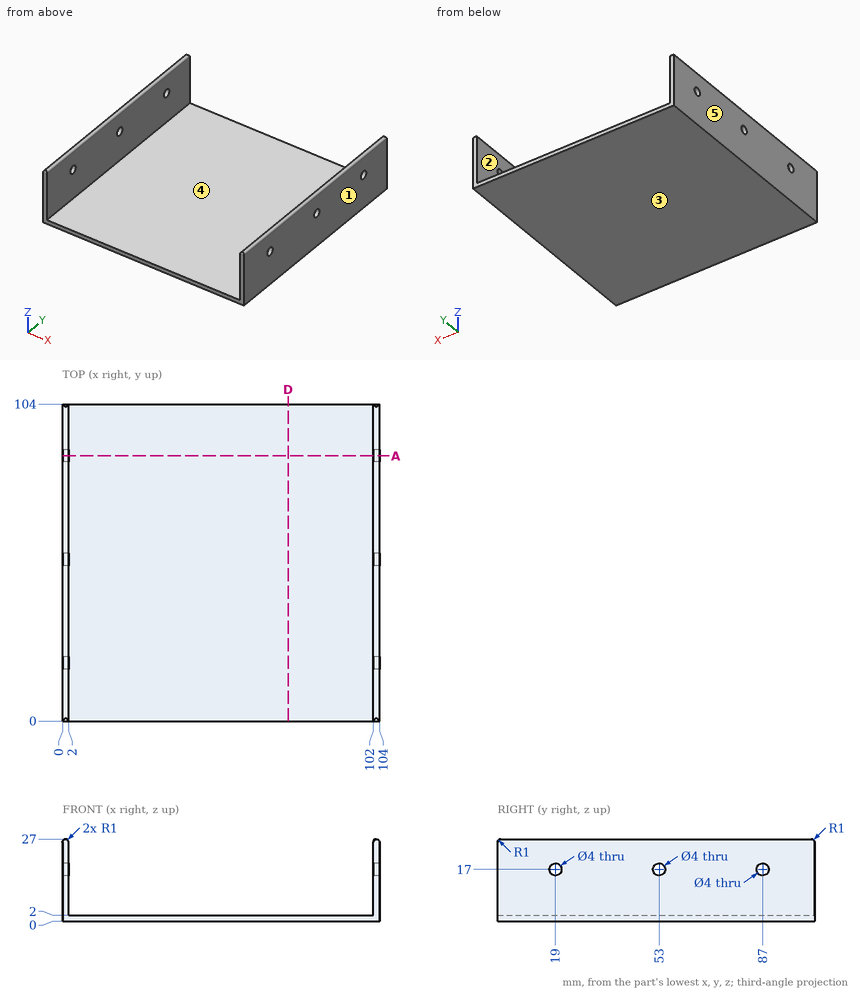
Answer from the drawing. Dimensions are ordinates in mm from the lowest x, y and z of the part. A direction names the side the tool comes from. Coordinates: 2 decimals unless noted, no trailing zeros. Write each loop counter-clockwise with the first axis right and the second up, starting at its lowest first coordinate (ties: lowest second). Pieces come first, ordered by that corner, then holes. Notation, with made-up numbers: (48.5, -39.5) - (92.5, -39.5) arc R24 cw to (92.5, -13.5) - close; hole circle Ø2 at (17.5, 65). An arc over 180 degrees is marked (long way). Return JSON: item names as keys, results as strings. Group by question number.
Q1. For a pull along X with two mould halves and no side action, classify the marked faces 3, 4 and 5 as +X half, -X half, draft (parallel to the pull), parting line (faces both ways), or undercut.
Q2. Find the intervals of material crossed by line 1 along X through (y, z) = (27, 23.5); line 2 along Z through (x, y) = (79, 39); line 3 along Z through (x, y) = (1.5, 87), in increasing order. Write a range as [from, to].
Q3. Which of the six approach directions +Z, -Z, +X, -X, +Y, -Y give full straight-line access (tool end or side, diameter ignored) to the marked faces 1 and 2?
Q4. Flat-ended cylindrical pins translate along their axes: pin 1 Ø2.5 at (y, z) = (87, 17) entering from +X; pin 2 Ø2 at (x, y) = (61.5, 48.5) entering from +Z. Find the tip coordinate at first contact, or state that the pin passes through.
Q5. The part is cut by section D-D on x = 74. Write down the section's boundary in (y, z), and give its area (3 significant figures).
Q6. The part is cut by section A-A on y = 87. State how many separate pieces and enclosed holes the cut face has, and give its area (3 significant figures).
Evaluation:
{
 "1": {"face 3": "draft", "face 4": "undercut", "face 5": "-X half"},
 "2": {"line 1": "x = [0, 2], [102, 104]", "line 2": "z = [0, 2]", "line 3": "z = [0, 15], [19, 26.87]"},
 "3": {"face 1": "+Z, -Z, +X, +Y, -Y", "face 2": "+Z, +Y, -Y"},
 "4": {"pin 1": "passes through", "pin 2": "stops at z = 2"},
 "5": {"outline": "(0, 0) - (104, 0) - (104, 2) - (0, 2) - close", "area": "208 mm2"},
 "6": {"separate pieces": "3", "enclosed holes": "0", "area": "291 mm2"}
}
